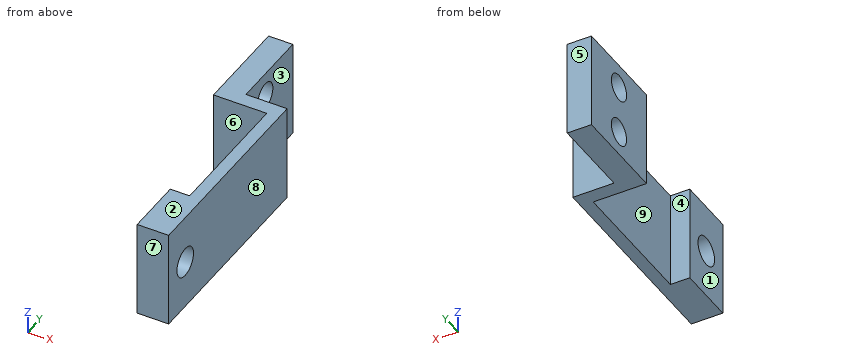
Autodesk Inventor part; units mm, degrees
ref_plane "YZ Plane" through (0, 0, 0) normal (1, 0, 0) x (0, 1, 0)
ref_plane "XZ Plane" through (0, 0, 0) normal (0, 1, 0) x (-1, 0, 0)
ref_plane "XY Plane" through (0, 0, 0) normal (0, 0, 1) x (1, 0, 0)
sketch "Sketch1" plane through (0, 0, 0) normal (1, 0, 0) x (0, 1, 0)
  line L0 (0, 0) -> (-26.6, 0)
  line L1 (-26.6, 0) -> (-26.6, -20)
  line L2 (-26.6, -20) -> (0, -20)
  line L3 (0, -20) -> (0, 0)
  line L4 (0, 0) -> (-10, 0) construction
  line L5 (-10, 0) -> (-10, -5) construction
  circle A0 centre (-10, -5) radius 2.75
  line L6 (0, -20) -> (-10, -20) construction
  line L7 (-10, -20) -> (-10, -15) construction
  circle A1 centre (-10, -15) radius 2.75
  line L8 (-26.6, 0) -> (-20, 0)
  line L9 (-20, 0) -> (-20, -20)
  line L10 (-20, -20) -> (-26.6, -20)
  line L11 (-26.6, -20) -> (-26.6, 0)
  line L12 (-20, 0) -> (-17, 0)
  line L13 (-17, 0) -> (-17, -20)
  line L14 (-17, -20) -> (-20, -20)
  line L15 (-20, -20) -> (-20, 0)
  dimension "d0" = 26.6
  dimension "d1" = 20
  dimension "d2" = 10
  dimension "d3" = 5
  dimension "d4" = 5.5
  dimension "d5" = 10
  dimension "d6" = 5
  dimension "d7" = 5.5
  dimension "d8" = 6.6
  dimension "d9" = 3
extrude "Extrusion1" add sketch "Sketch1" along normal blind 8.5 contours L13 L2 L9 L0
extrude "Extrusion2" add sketch "Sketch1" against normal blind 5 contours L3 L2 L13 L0
extrude "Extrusion3" add sketch "Sketch1" against normal blind 5 contours L13 L2 L9 L0
sketch "Sketch2" plane through (8.5, -20, -20) normal (0, -1, 0) x (1, 0, 0)
  line L0 (0, 20) -> (0, 0)
  line L1 (-8.5, 0) -> (0, 0)
  line L2 (0, 20) -> (-2.5, 20)
  line L3 (-2.5, 20) -> (-2.5, 0)
  line L4 (-2.5, 0) -> (0, 0)
  line L5 (0, 0) -> (0, 20)
  point P0 (-8.5, 20)
  dimension "d16" = 2.5
extrude "Extrusion4" add sketch "Sketch2" along normal blind 40
sketch "Sketch3" plane through (8.5, 0, 0) normal (1, 0, 0) x (0, 0, -1)
  line L0 (20, -60) -> (0, -60)
  circle A0 centre (10, -54) radius 3
  point P0 (0, 0)
  dimension "d20" = 6
extrude "Extrusion5" cut sketch "Sketch3" against normal blind 7.5
sketch "Sketch4" plane through (6, -20, -20) normal (-1, 0, 0) x (0, 0, 1)
  line L0 (20, 3) -> (20, -40)
  line L1 (0, 3) -> (0, -40)
  line L2 (20, -40) -> (0, -40)
  line L3 (0, -40) -> (0, -28)
  line L4 (0, -28) -> (20, -28)
  line L5 (20, -28) -> (20, -40)
  point P0 (20, 20)
  dimension "d23" = 12
extrude "Extrusion6" add sketch "Sketch4" along normal blind 4
sketch "Sketch5" plane through (6, -54, -10) normal (1, 0, 0) x (0, 0, -1)
  circle A0 centre (0, 0) radius 3
  point P0 (-10, 54)
extrude "Extrusion7" cut sketch "Sketch5" against normal blind 4
properties part number "Laser_Holder"
Could you check a few things on this model? Use its own coordinates, in mm. Face numbers are marked on the shaded views. A direction names the side the tool comes from. Coordinates: 2 decimals unless noted, no trailing zeros. Order: outer loops, then holes, each group sorted by start corner. A loop starts at its lowest first (then second) coordinate and runs counter-clockwise, first axis right, second up. Notation, with made-up numbers: (-7.75, 39.5) -> (43.25, 39.5) arc R15 cw to (43.25, 55.5) -> close; hole circle Ø8 at (47, 32). An arc over 180 degrees is marked (long way). One line per item, written item: value. Start each with the question number.
1) Imagine slicing it at B-B on y = -54. List the corners of the cut face in (x, z) for me, plus the area to 3 significant figures.
2) Imagine slicing it at A-A on z = -10. List the corners of the cut face in (x, y) for me.
3) I'm going to push flat-ended pins straight in: pin 1 (3.5 mm diameter, centred on x = -2, z = -15, fed in from -Y); pin 2 (7 mm diameter, centred on y = -54, z = -10, fed in from +X); pin 3 (3 mm diameter, centred on x = 4, z = -10, fed in from +Y); pin 4 (5 mm diameter, centred on y = -27.5, z = -7, fed in from -X). Where does each tip first touch, or does it pass through?
4) If I drill on L1, parallel to Y at x = 4.75, z = -10; L2, parallel to Z at x = -3.35, y = -10; L3, parallel to Y at x = 5.5, z = -14.5, over which ranges is the centre line in solid material (lowest first)? Write a range as [from, to].
5) Imagine slicing it at C-C on y = -10. List the corners of the cut face in (x, z) for me, plus the area to 3 significant figures.
6) We'd pull the mould along Y, two halves only. Please class the marked faces 6, 7, 8 and 9: +Y half, -Y half, draft (parallel to the pull), parting line (faces both ways), or undercut.
7) Imagine slicing it at D-D on z = -5. List the corners of the cut face in (x, y) for me, plus the area to 3 significant figures.
8) Which directions (+Z, -Z, +X, -X, +Y, -Y) give clear straight access to the entire face, cutting with the end or side of a thin tool? Please do the marked faces 1, 2, 3, 4 and 5.
Answer list:
1. outline: (2, -20) -> (8.5, -20) -> (8.5, -13) -> (2, -13) -> close; (2, -7) -> (8.5, -7) -> (8.5, 0) -> (2, 0) -> close
1. area: 91.0 mm2
2. outline: (-5, -20) -> (6, -20) -> (6, -48) -> (2, -48) -> (2, -51) -> (8.5, -51) -> (8.5, -17) -> (0, -17) -> (0, 0) -> (-5, 0) -> close; (2, -60) -> (8.5, -60) -> (8.5, -57) -> (2, -57) -> close
3. pin 1: stops at y = -20
3. pin 2: stops at x = 8.5
3. pin 3: stops at y = -17
3. pin 4: stops at x = 6
4. L1: y = [-60, -57], [-51, -48], [-20, -17]
4. L2: z = [-20, -17.75], [-12.25, -7.75], [-2.25, 0]
4. L3: y = [-60, -48], [-20, -17]
5. outline: (-5, -20) -> (0, -20) -> (0, -17.75) -> (-5, -17.75) -> close; (-5, -12.25) -> (0, -12.25) -> (0, -7.75) -> (-5, -7.75) -> close; (-5, -2.25) -> (0, -2.25) -> (0, 0) -> (-5, 0) -> close
5. area: 45.0 mm2
6. face 6: undercut
6. face 7: -Y half
6. face 8: draft
6. face 9: undercut
7. outline: (-5, -20) -> (6, -20) -> (6, -48) -> (2, -48) -> (2, -60) -> (8.5, -60) -> (8.5, -17) -> (0, -17) -> (0, -12.75) -> (-5, -12.75) -> close; (-5, -7.25) -> (0, -7.25) -> (0, 0) -> (-5, 0) -> close
7. area: 246 mm2
8. face 1: +Z, -Z, -X, -Y
8. face 2: +Z, +X, -X, +Y, -Y
8. face 3: +Z, -Z, +X, +Y
8. face 4: +Z, -Z, -X
8. face 5: +Z, -Z, +X, -X, +Y
